Model file for the job. Use its own axes, mm. Face numbers are marked on the shaded views. Coordinates: 2 decimals unless noted, no trailing zeros. Order: outer loops, then holes, each group sorted by start corner. A loop starts at its lowest first (then second) coordinate and runs counter-clockwise, first axis right, second up. Notation, with made-up numbers: (83, 52.25) -> (89, 52.25) arc R19 cw to (89, 69.25) -> close; hole circle Ø6 at (77, 11.25). An arc over 180 degrees is marked (long way). Return JSON: item names as keys, results as strings. Group by question number.
1) Cut at D-D (z = 48.5). Write the cut outline in (x, y).
2) Probe line 1 (Y direction, x = 12.5, z = 37); line 2 (Z direction, x = 16.5, y = -74.5); line 3 (Z direction, x = 3.5, y = 28.5). List the from-to ranges inside material, lowest first.
3) Flat gauge pins, fed straight in: pin 1 (10 mm diameter, centred on x = 4, z = -30, fed in from +Y); pin 2 (4 mm diameter, centred on x = 10.5, z = 65, fed in from +Y); pin 3 (8 mm diameter, centred on x = 16.5, z = -31, fed in from +Y). Where does each tip first touch, or does it go through?
4) Pull direction Y, two halves, no side cores. Call the marked faces 1, 2 and 3: +Y half, -Y half, draft (parallel to the pull), parting line (faces both ways), or undercut.
5) Cut at C-C (x = 13.5). State how many separate pieces and enclosed holes the cut face has, and give its area (3 significant figures).
6) Cut at A-A (y = 0). Write the cut outline in (x, z).
Autodesk Inventor part; units mm, degrees
ref_plane "YZ Plane" through (0, 0, 0) normal (1, 0, 0) x (0, 1, 0)
ref_plane "XZ Plane" through (0, 0, 0) normal (0, 1, 0) x (-1, 0, 0)
ref_plane "XY Plane" through (0, 0, 0) normal (0, 0, 1) x (1, 0, 0)
sketch "Sketch1" plane through (0, 0, 0) normal (0, 0, 1) x (1, 0, 0)
  line L0 (20, 100) -> (0, 100)
  line L1 (0, 100) -> (0, 45.25)
  line L2 (0, 45.25) -> (0, 0) construction
  line L3 (0, 0) -> (20, 0) construction
  line L4 (20, 100) -> (20, 45.25)
  line L5 (20, 45.25) -> (0, 45.25)
  line L6 (20, 45.25) -> (20, 0) construction
  dimension "d0" = 200
  dimension "d1" = 20
  dimension "d6" = 90.5
revolve "Revolution1" add sketch "Sketch1" angle 360 about axis through (0, 0, 0) along (1, 0, 0)
sketch "Sketch2" plane through (0, 0, 0) normal (-1, 0, 0) x (0, 0, 1)
  circle A0 centre (0, 0) radius 45.25
  circle A1 centre (0, 0) radius 80 construction
  line L0 (0, 80) -> (0, 0) construction
  circle A2 centre (0, 0) radius 100
  circle A3 centre (30.6147, 73.9104) radius 9
  line L1 (0, 0) -> (30.6147, 73.9104) construction
  dimension "d2" = 160
  dimension "d7" = 18
  dimension "d8" = 22.5
extrude "Extrusion1" cut sketch "Sketch2" against normal through all contours A3
pattern_circular "Circular Pattern1" count 8 over 360 about axis through (10, 0, 0) along (1, 0, 0) of "Extrusion1"
equation "\"d0\" = D"
equation "\"d1\" = C1"
equation "\"d6\" = B1"
equation "\"d2\" = K1"
equation "\"d7\" = L"
equation "\"C1\" = 20"
equation "\"D\" = 200"
equation "\"K1\" = 160"
equation "\"L\" = 18"
equation "\"B1\" = 90.5"
equation "\"NB\" = 1.2345"
equation "\"Size_Designation\" = 1.2345"
properties part number "ISO 7005-1 Plate Flange for Welding Type 01 Flat Face - ISO PN 16 DN80" material "Steel"
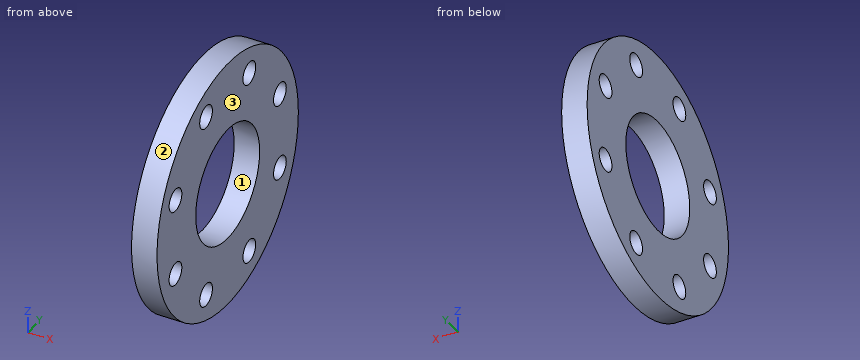
Answers below:
{
 "1": {"outline": "(0, -87.45) -> (20, -87.45) -> (20, 87.45) -> (0, 87.45) -> close"},
 "2": {"line 1": "y = -92.9 to -80.25, -67.57 to -26.05, 26.05 to 67.57, 80.25 to 92.9", "line 2": "z = -66.71 to -39.6, -21.63 to 21.63, 39.6 to 66.71", "line 3": "z = -95.85 to -82.66, -65.16 to -35.15, 35.15 to 65.16, 82.66 to 95.85"},
 "3": {"pin 1": "stops at y = 96.82", "pin 2": "stops at y = 77.66", "pin 3": "stops at y = 96.29"},
 "4": {"face 1": "undercut", "face 2": "parting line", "face 3": "draft"},
 "5": {"separate pieces": "1", "enclosed holes": "9", "area": "22,900 mm^2"},
 "6": {"outline": "(0, -100) -> (20, -100) -> (20, -45.25) -> (0, -45.25) -> close; (0, 45.25) -> (20, 45.25) -> (20, 100) -> (0, 100) -> close"}
}
